The drawing under review shows one solid part. Ordinate dimensions are in mm from its lowest x, y, z. A direction names the side the tool comes from. Give positions to 0.01 mm unless a question says otherwise; leave off trailing zeros. Write each loop counter-clockwise with the first axis right and the second up, starting at its lowest first coordinate (ties: lowest second). Pieces come first, ordered by that corner, then holes. Notation, with made-up numbers: (86, 83) -> (95, 83) arc R16 cw to (95, 87) -> close; hole circle Ø6 at (31.25, 13). An arc over 180 degrees is marked (long way). Answer as a JSON object with one key per item and string values.
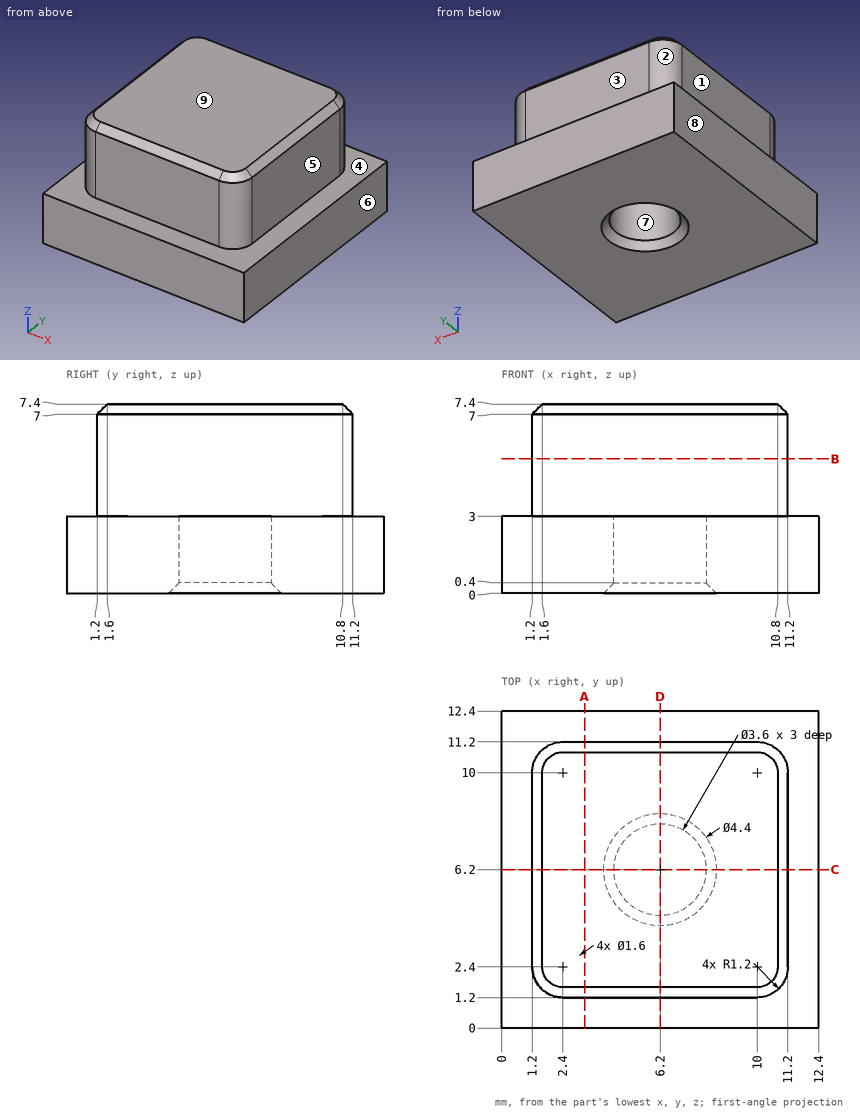
(1) We need section B-B, the plane z = 5.25. State the section outline as (x, y) points.
Here are the results:
{"outline": "(1.2, 2.4) arc R1.2 ccw to (2.4, 1.2) -> (10, 1.2) arc R1.2 ccw to (11.2, 2.4) -> (11.2, 10) arc R1.2 ccw to (10, 11.2) -> (2.4, 11.2) arc R1.2 ccw to (1.2, 10) -> close"}
(2) We need section A-A, the plane x = 3.25. State the section outline as (y, z) points, then the cut area to 3 significant figures.
Here are the results:
{"outline": "(0, 0) -> (12.4, 0) -> (12.4, 3) -> (11.2, 3) -> (11.2, 7) -> (10.8, 7.4) -> (1.6, 7.4) -> (1.2, 7) -> (1.2, 3) -> (0, 3) -> close", "area": "81.0 mm²"}
(3) The part is to be moulded in two halves that separate along X. For the marked faces 6, 7, 8 and 9, say which applies: +X half, -X half, draft (parallel to the pull), parting line (faces both ways), or undercut.
Here are the results:
{"face 6": "+X half", "face 7": "undercut", "face 8": "-X half", "face 9": "draft"}
(4) For line 1 along Y through (x, z) = (6.2, 2.5); line 2 along X through (y, z) = (7, 2); line 3 along Z through (x, y) = (11.75, 11.25), list the stretches that pass through material, from the lowest coordinate up.
Here are the results:
{"line 1": "y = 0 to 4.4, 8 to 12.4", "line 2": "x = 0 to 4.59, 7.81 to 12.4", "line 3": "z = 0 to 3"}
(5) We need section C-C, the plane y = 6.2. State the section outline as (x, z) points.
Here are the results:
{"outline": "(0, 0) -> (4, 0) -> (4.4, 0.4) -> (4.4, 3) -> (8, 3) -> (8, 0.4) -> (8.4, 0) -> (12.4, 0) -> (12.4, 3) -> (11.2, 3) -> (11.2, 7) -> (10.8, 7.4) -> (1.6, 7.4) -> (1.2, 7) -> (1.2, 3) -> (0, 3) -> close"}
(6) For the marked faces 1, 2, 3, 4 and 5, list the 3-axis set-ups (+Z, -Z, +X, -X, +Y, -Y) from which the entire face can be reached by the end or side of a thin tool; tool diameter is ignored.
Here are the results:
{"face 1": "+Z, -X, +Y, -Y", "face 2": "+Z, -X, +Y", "face 3": "+Z, +X, -X, +Y", "face 4": "+Z", "face 5": "+Z, +X, +Y, -Y"}
(7) Clearance check with flat-ended pins moving along their axes: pin 1 (3 mm diameter, centred on x = 4.5, z = 5.5, fed in from +Y); pin 2 (1.2 mm diameter, centred on x = 7, z = 4.5, fed in from -Y); pin 3 (1.1 mm diameter, centred on x = 6, y = 6.5, fed in from -Z). State where each tip first meets the part, or that it passes through.
Here are the results:
{"pin 1": "stops at y = 11.2", "pin 2": "stops at y = 1.2", "pin 3": "stops at z = 3"}
